Source: CAD feature listing. Evaluate the final solid. Frame: model axes, mm. A direction names the side the tool comes from. Round coordinates to 2 decimals unless told otherwise and drop trailing zeros. Write each loop counter-clockwise with the first axis right and the second up, starting at its lowest first coordinate (ties: lowest second). Pieces come first, ordered by that corner, then holes. Notation, with made-up numbers: M 2.5,83 L 61.5,83 A21 ccw 61.5,90 Z; hole C 23.5,-14 d11. An arc over 180 degrees is marked long. Use a Markdown table: item, result.
```python
from build123d import *

# Parameters (mm, degrees)
F0_R     = 2.5
F1_DEPTH = 3.175


with BuildPart() as f1:
    # F0 (on Top) → F1 (new body)
    with BuildSketch(Plane.XY):
        with BuildLine():
            Line((-69.85, 12.7), (-76.2, 12.7))
            Line((-76.2, 12.7), (-76.2, -12.7))
            Line((-76.2, -12.7), (-69.85, -12.7))
            Line((-69.85, -12.7), (-67.945, -12.7))
            Line((-67.945, -12.7), (-67.945, -15.875))
            Line((-67.945, -15.875), (-55.245, -15.875))
            Line((-55.245, -15.875), (-55.245, -12.7))
            Line((-55.245, -12.7), (-53.34, -12.7))
            Line((-53.34, -12.7), (-34.29, -12.7))
            Line((-34.29, -12.7), (-32.385, -12.7))
            Line((-32.385, -12.7), (-32.385, -15.875))
            Line((-32.385, -15.875), (-19.685, -15.875))
            Line((-19.685, -15.875), (-19.685, -12.7))
            Line((-19.685, -12.7), (62.480263, -12.7))
            Line((62.480263, -12.7), (63.47136, -12.7))
            Line((63.47136, -12.7), (88.92864, -12.7))
            Line((88.92864, -12.7), (89.919737, -12.7))
            Line((89.919737, -12.7), (93.133333, -12.7))
            ThreePointArc((93.133333, -12.7), (99.120171, -10.220171), (101.6, -4.233333))
            Line((101.6, -4.233333), (101.6, 4.233333))
            ThreePointArc((101.6, 4.233333), (99.120171, 10.220171), (93.133333, 12.7))
            Line((93.133333, 12.7), (76.2, 12.7))
            Line((76.2, 12.7), (-19.685, 12.7))
            Line((-19.685, 12.7), (-19.685, 15.875))
            Line((-19.685, 15.875), (-32.385, 15.875))
            Line((-32.385, 15.875), (-32.385, 12.7))
            Line((-32.385, 12.7), (-34.29, 12.7))
            Line((-34.29, 12.7), (-53.34, 12.7))
            Line((-53.34, 12.7), (-55.245, 12.7))
            Line((-55.245, 12.7), (-55.245, 15.875))
            Line((-55.245, 15.875), (-67.945, 15.875))
            Line((-67.945, 15.875), (-67.945, 12.7))
            Line((-67.945, 12.7), (-69.85, 12.7))
        make_face()
        with Locations((76.2, 0)):
            Circle(F0_R, mode=Mode.SUBTRACT)
    extrude(amount=F1_DEPTH)


solid = f1.part
```
Q1. Mould query, pull axis X, two halves, no side actions, for faces 1 (the flat face through (-26, 15.875, 2)), 2 (the cylindrical face through (99.19, 10.15, 1.57)), 3 (the flat face through (-32.385, -14, 2)), 4 (the flat face through (-44, -12.7, 2)). Classes: +X half, -X half, draft (parallel to the pull), parting line (faces both ways), or undercut.
Results are:
| item | result |
|---|---|
| face 1 | draft |
| face 2 | +X half |
| face 3 | undercut |
| face 4 | undercut |
Q2. Section A-A on x = 76.2. Return loops of the section in (y, z) (3 decimals).
Results are:
| item | result |
|---|---|
| outline | M -12.7,0 L -2.5,0 L -2.5,3.175 L -12.7,3.175 Z; M 2.5,0 L 12.7,0 L 12.7,3.175 L 2.5,3.175 Z |
Q3. First-contact query: pin 1 Ø1.5 at (x, z) = (10.5, 2.5) entering from +Y; pin 2 Ø1.6 at (x, z) = (-74, 1) entering from -Y; pin 3 Ø1 at (y, z) = (13.5, 2) entering from -X (3 decimals). Flat tips, straight axial feed; report the tip coordinate or a pass-through.
Results are:
| item | result |
|---|---|
| pin 1 | y = 12.7 |
| pin 2 | y = -12.7 |
| pin 3 | x = -67.945 |
Q4. Line query: L1, parallel to Y at x = 76.2, z = 2.25; L2, parallel to X at y = -14, z = 1.15 (3 decimals); L3, parallel to Y at x = 14.5, z = 1.95. Output: solid intervals per line, ascending.
Results are:
| item | result |
|---|---|
| L1 | -12.7 to -2.5, 2.5 to 12.7 |
| L2 | -67.945 to -55.245, -32.385 to -19.685 |
| L3 | -12.7 to 12.7 |
Q5. Reachability of faces 5 (the flat face through (-72, -12.7, 2)), 6 (the flat face through (-55.245, -14, 2)), 7 (the flat face through (-19.685, -14, 2)), 8 (the flat face through (-19.685, 14, 2)), 9 (the flat face through (-55.245, 14, 2)) from +Z, -Z, +X, -X, +Y, -Y: full face, straight path, thin tool, end or side. Return the list, or none.
Results are:
| item | result |
|---|---|
| face 5 | +Z, -Z, -X, -Y |
| face 6 | +Z, -Z, -Y |
| face 7 | +Z, -Z, +X, -Y |
| face 8 | +Z, -Z, +X, +Y |
| face 9 | +Z, -Z, +Y |
Q6. Section C-C on z = 0.6. Return loops of the section in (x, y) (3 decimals).
Results are:
| item | result |
|---|---|
| outline | M -76.2,-12.7 L -67.945,-12.7 L -67.945,-15.875 L -55.245,-15.875 L -55.245,-12.7 L -32.385,-12.7 L -32.385,-15.875 L -19.685,-15.875 L -19.685,-12.7 L 93.133,-12.7 A8.467 ccw 101.6,-4.233 L 101.6,4.233 A8.467 ccw 93.133,12.7 L -19.685,12.7 L -19.685,15.875 L -32.385,15.875 L -32.385,12.7 L -55.245,12.7 L -55.245,15.875 L -67.945,15.875 L -67.945,12.7 L -76.2,12.7 Z; hole C 76.2,0 d5 |
Q7. Section D-D on x = -6. Return loops of the section in (y, z) (3 decimals).
Results are:
| item | result |
|---|---|
| outline | M -12.7,0 L 12.7,0 L 12.7,3.175 L -12.7,3.175 Z |
Q8. Section B-B on y = 0. Return loops of the section in (x, z) (3 decimals).
Results are:
| item | result |
|---|---|
| outline | M -76.2,0 L 73.7,0 L 73.7,3.175 L -76.2,3.175 Z; M 78.7,0 L 101.6,0 L 101.6,3.175 L 78.7,3.175 Z |
